Read the model definition and answer for the solid it produces. Units are mm, in the model's axes. Face numbers are marked on the shaded views. A direction names the side the tool comes from. Give positions to 0.01 mm unless a question says otherwise; leave off trailing zeros. Write each loop counter-clockwise with the first axis right and the second up, starting at its lowest first coordinate (ties: lowest second). Pieces come first, ordered by that corner, then holes. Notation, with made-up numbers: M 37,44 L 57,44 A31 cw 57,72 Z; hole C 50,30 d8. An arc over 180 degrees is marked long. Put each result on its own line as item: value.
from build123d import *

# Parameters (mm, degrees)
ESQUISSE1_R        = 4
ESQUISSE1_R_2      = 1.59999944
BOSS_EXTRU_1_DEPTH = 5


with BuildPart() as part:
    # Esquisse1 → Boss.-Extru.1 (new body)
    with BuildSketch(Plane(origin=(0, 0, 0), x_dir=(-1, 0, 0), z_dir=(0, 0, -1))):
        with BuildLine():
            Line((-8.039665, 5.193958), (-7.511682, 7.163724))
            Line((-7.511682, 7.163724), (-6.637512, 8.89434))
            Line((-6.637512, 8.89434), (-5.734358, 10.21466))
            Line((-5.734358, 10.21466), (-4.529502, 11.42329))
            Line((-4.529502, 11.42329), (-3.426544, 12.65958))
            Line((-3.426544, 12.65958), (-2.422703, 14.23997))
            Line((-2.422703, 14.23997), (-1.578115, 16.23473))
            Line((-1.578115, 16.23473), (-0.7880442, 19.27814))
            Line((-0.7880442, 19.27814), (-0.2469295, 23.26466))
            Line((-0.2469295, 23.26466), (-0.008147676, 28.26909))
            Line((-0.008147676, 28.26909), (0, 29.5))
            Line((0, 29.5), (-0.01509115, 31.16446))
            Line((-0.01509115, 31.16446), (-0.2937396, 36.23574))
            Line((-0.2937396, 36.23574), (-0.8642389, 40.10257))
            Line((-0.8642389, 40.10257), (-1.681502, 43.05889))
            Line((-1.681502, 43.05889), (-2.667923, 45.20577))
            Line((-2.667923, 45.20577), (-3.68381, 46.66188))
            Line((-3.68381, 46.66188), (-5.121313, 48.15284))
            Line((-5.121313, 48.15284), (-6.221777, 49.42276))
            Line((-6.221777, 49.42276), (-7.084233, 50.913))
            Line((-7.084233, 50.913), (-7.705722, 52.38649))
            Line((-7.705722, 52.38649), (-8.155009, 54.60259))
            Line((-8.155009, 54.60259), (-8.534575, 55.99675))
            Line((-8.534575, 55.99675), (-9.29695, 57.22417))
            Line((-9.29695, 57.22417), (-10.37847, 58.18233))
            Line((-10.37847, 58.18233), (-11.68882, 58.79123))
            Line((-11.68882, 58.79123), (-13.11856, 59))
            Line((-13.11856, 59), (-28.5, 59))
            ThreePointArc((-28.5, 59), (-28.853553391, 58.853553391), (-29, 58.5))
            Line((-29, 58.5), (-29, 54.25))
            Line((-29, 54.25), (-28.875, 54.2165))
            Line((-28.875, 54.2165), (-28.78349, 54.125))
            Line((-28.78349, 54.125), (-28.75, 54))
            Line((-28.75, 54), (-28.78349, 53.875))
            Line((-28.78349, 53.875), (-28.875, 53.78349))
            Line((-28.875, 53.78349), (-29, 53.75))
            Line((-29, 53.75), (-29.125, 53.78349))
            Line((-29.125, 53.78349), (-29.21651, 53.875))
            Line((-29.21651, 53.875), (-29.25, 54))
            Line((-29.25, 54), (-33.75, 54))
            ThreePointArc((-33.75, 54), (-34.176776695, 53.823223305), (-34, 54.25))
            Line((-34, 54.25), (-34, 58.5))
            ThreePointArc((-34, 58.5), (-34.146446609, 58.853553391), (-34.5, 59))
            Line((-34.5, 59), (-34.77157, 59))
            Line((-34.77157, 59), (-35.53694, 58.84776))
            Line((-35.53694, 58.84776), (-36.18579, 58.41422))
            Line((-36.18579, 58.41422), (-39.41421372, 55.18578628))
            ThreePointArc((-39.41421372, 55.18578628), (-39.847759129, 54.53693809), (-40, 53.77157))
            Line((-40, 53.77157), (-40, 5.228428))
            ThreePointArc((-40, 5.228428), (-39.847759811, 4.463063957), (-39.414216379, 3.814219379))
            Line((-39.414216379, 3.814219379), (-36.18579, 0.585787))
            ThreePointArc((-36.18579, 0.585787), (-35.536943679, 0.152241095), (-34.771576938, 0))
            Line((-34.771576938, 0), (-17.5, 0))
            ThreePointArc((-17.5, 0), (-17.146446609, 0.146446609), (-17, 0.5))
            Line((-17, 0.5), (-17, 4.75))
            Line((-17, 4.75), (-17.125, 4.783494))
            Line((-17.125, 4.783494), (-17.21651, 4.875))
            Line((-17.21651, 4.875), (-17.25, 5.000001))
            Line((-17.25, 5.000001), (-17.21651, 5.125001))
            Line((-17.21651, 5.125001), (-17.125, 5.216507))
            Line((-17.125, 5.216507), (-17, 5.25))
            Line((-17, 5.25), (-16.875, 5.216507))
            Line((-16.875, 5.216507), (-16.78349, 5.125001))
            Line((-16.78349, 5.125001), (-16.75, 5.000001))
            Line((-16.75, 5.000001), (-12.25, 5.000001))
            Line((-12.25, 5.000001), (-12.21651, 5.125001))
            Line((-12.21651, 5.125001), (-12.125, 5.216507))
            Line((-12.125, 5.216507), (-12, 5.25))
            Line((-12, 5.25), (-11.875, 5.216507))
            Line((-11.875, 5.216507), (-11.78349, 5.125001))
            Line((-11.78349, 5.125001), (-11.75, 5.000001))
            Line((-11.75, 5.000001), (-11.78349, 4.810393211))
            Line((-11.78349, 4.810393211), (-11.875, 4.718887211))
            Line((-11.875, 4.718887211), (-12, 4.685393211))
            Line((-12, 4.685393211), (-12, 0.500001))
            ThreePointArc((-12, 0.500001), (-11.853553098, 0.146446902), (-11.499999, 0))
            Line((-11.499999, 0), (-10.33203, 0))
            Line((-10.33203, 0), (-9.352249, 0.2564304))
            Line((-9.352249, 0.2564304), (-8.623715, 0.9599663))
            Line((-8.623715, 0.9599663), (-8.333246, 1.9302))
            Line((-8.333246, 1.9302), (-8.039665, 5.193958))
        make_face()
        with Locations((-23, 52)):
            Circle(ESQUISSE1_R, mode=Mode.SUBTRACT)
        with Locations((-23, 6.999999)):
            Circle(ESQUISSE1_R, mode=Mode.SUBTRACT)
        with Locations((-7, 29.499999)):
            Circle(ESQUISSE1_R_2, mode=Mode.SUBTRACT)
        with BuildLine():
            Line((-27.85382, 44.42105), (-25.78795, 43.4427))
            Line((-25.78795, 43.4427), (-23.54223, 43.01635))
            Line((-23.54223, 43.01635), (-21.26154, 43.1695))
            Line((-21.26154, 43.1695), (-19.09299, 43.89227))
            Line((-19.09299, 43.89227), (-17.17647, 45.13804))
            Line((-17.17647, 45.13804), (-17.04626, 45.30922))
            Line((-17.04626, 45.30922), (-17, 45.51926))
            Line((-17, 45.51926), (-17, 50.75))
            ThreePointArc((-17, 50.75), (-17.176776695, 51.176776695), (-16.75, 51))
            Line((-16.75, 51), (-12.25, 51))
            ThreePointArc((-12.25, 51), (-11.823223305, 51.176776695), (-12, 50.75))
            Line((-12, 50.75), (-12, 46.412623211))
            Line((-12, 46.412623211), (-11.9404, 46.175873211))
            Line((-11.9404, 46.175873211), (-11.7758, 45.995563211))
            Line((-11.7758, 45.995563211), (-11.54545, 45.914693211))
            Line((-11.54545, 45.914693211), (-10.113, 45.565643211))
            Line((-10.113, 45.565643211), (-8.844621, 44.813993211))
            Line((-8.844621, 44.813993211), (-7.850602, 43.725103211))
            Line((-7.850602, 43.725103211), (-7.217376, 42.393653211))
            Line((-7.217376, 42.393653211), (-7, 40.935393211))
            Line((-7, 40.935393211), (-7.619118173, 39.531113076))
            Line((-7.619118173, 39.531113076), (-8.678014173, 38.335053076))
            Line((-8.678014173, 38.335053076), (-10.060093173, 37.534003076))
            Line((-10.060093173, 37.534003076), (-12.077863173, 36.434693076))
            Line((-12.077863173, 36.434693076), (-13.732523173, 34.840353076))
            Line((-13.732523173, 34.840353076), (-14.905963173, 32.864763076))
            Line((-14.905963173, 32.864763076), (-15.514393173, 30.648993076))
            Line((-15.514393173, 30.648993076), (-15.514393173, 28.351193076))
            Line((-15.514393173, 28.351193076), (-14.905963173, 26.135413076))
            Line((-14.905963173, 26.135413076), (-13.732523173, 24.159833076))
            Line((-13.732523173, 24.159833076), (-12.077863173, 22.565493076))
            Line((-12.077863173, 22.565493076), (-10.060093173, 21.466183076))
            Line((-10.060093173, 21.466183076), (-8.678014173, 20.665133076))
            Line((-8.678014173, 20.665133076), (-7.619118173, 19.469073076))
            Line((-7.619118173, 19.469073076), (-6.991483173, 18.000093076))
            Line((-6.991483173, 18.000093076), (-7.244718, 16.45492))
            Line((-7.244718, 16.45492), (-7.954915, 15.06107))
            Line((-7.954915, 15.06107), (-9.061074, 13.95492))
            Line((-9.061074, 13.95492), (-10.45492, 13.24472))
            Line((-10.45492, 13.24472), (-12, 13))
            Line((-12, 13), (-16.0718, 13))
            Line((-16.0718, 13), (-16.27048, 13.04117))
            Line((-16.27048, 13.04117), (-16.43644, 13.1579))
            Line((-16.43644, 13.1579), (-18.19056, 14.60719))
            Line((-18.19056, 14.60719), (-20.2521, 15.57024))
            Line((-20.2521, 15.57024), (-22.48927, 15.9855))
            Line((-22.48927, 15.9855), (-24.7591, 15.82641))
            Line((-24.7591, 15.82641), (-26.91648, 15.10316))
            Line((-26.91648, 15.10316), (-28.82353, 13.86196))
            Line((-28.82353, 13.86196), (-28.95374, 13.69078))
            Line((-28.95374, 13.69078), (-29, 13.48074))
            Line((-29, 13.48074), (-29, 8.25))
            Line((-29, 8.25), (-28.875, 8.216506))
            Line((-28.875, 8.216506), (-28.78349, 8.125))
            Line((-28.78349, 8.125), (-28.75, 8))
            Line((-28.75, 8), (-28.78349, 7.875001))
            Line((-28.78349, 7.875001), (-28.875, 7.783493))
            Line((-28.875, 7.783493), (-29, 7.750001))
            Line((-29, 7.750001), (-29.125, 7.783493))
            Line((-29.125, 7.783493), (-29.21651, 7.875001))
            Line((-29.21651, 7.875001), (-29.25, 8))
            Line((-29.25, 8), (-33.75, 8))
            Line((-33.75, 8), (-33.7835, 7.875001))
            Line((-33.7835, 7.875001), (-33.875, 7.783493))
            Line((-33.875, 7.783493), (-34, 7.750001))
            Line((-34, 7.750001), (-34.125, 7.783493))
            Line((-34.125, 7.783493), (-34.21651, 7.875001))
            Line((-34.21651, 7.875001), (-34.25, 8))
            Line((-34.25, 8), (-34.21651, 8.125))
            Line((-34.21651, 8.125), (-34.125, 8.216506))
            Line((-34.125, 8.216506), (-34, 8.25))
            Line((-34, 8.25), (-34, 43.90222))
            Line((-34, 43.90222), (-33.81641, 44.73928))
            Line((-33.81641, 44.73928), (-33.29933, 45.42266))
            Line((-33.29933, 45.42266), (-32.54371, 45.8269))
            Line((-32.54371, 45.8269), (-31.68826, 45.87778))
            Line((-31.68826, 45.87778), (-29.69555, 45.34813))
            Line((-29.69555, 45.34813), (-27.85382, 44.42105))
        make_face(mode=Mode.SUBTRACT)
    extrude(amount=-BOSS_EXTRU_1_DEPTH)


solid = part.part
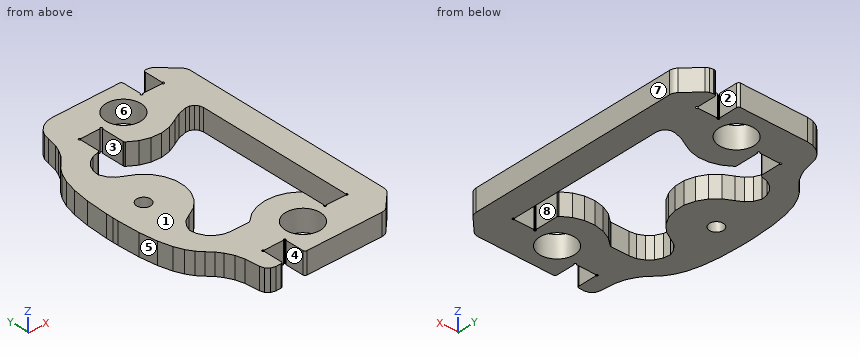
(1) Section A-A on y = 34 is taken. Determine the outline of the cut face in (x, z).
Result:
outline: M 0.17,0 L 14.23,0 L 14.23,5 L 0.17,5 Z; M 34,0 L 40,0 L 40,5 L 34,5 Z
(2) Which of the six approach directions +Z, -Z, +X, -X, +Y, -Y give full straight-line access (tool end or side, diameter ignored) to the marked faces 1, 2, 3 and 4?
Result:
face 1: +Z, +X, -X, +Y, -Y
face 2: +Z, -Z, +Y
face 3: +Z, -Z
face 4: +Z, -Z, -Y
(3) Section B-B on z = 3 is taken. Give the number of separate pieces and of enclosed holes in the cut face, and give its area (3 significant figures).
Result:
separate pieces: 1
enclosed holes: 4
area: 1,210 mm²
(4) Given pin 1 Ø1.3 at (x, z) = (15, 1.5) entering from -Y; pin 2 Ø1.3 at (y, z) = (2, 2.5) entering from -X; pin 3 Ø2 at (y, z) = (57, 2) entering from +X; pin 4 Ø5 at (x, y) = (23, 7) entering from -Z, each flat-ended and moving along its own axis, determine where each tip first touches the part or whether it passes through.
Result:
pin 1: stops at y = 5
pin 2: stops at x = 8.27
pin 3: stops at x = 38.6
pin 4: passes through
(5) For a pull along X with two mould halves and no side action, classify the marked faces 5, 6, 7 and 8 as +X half, -X half, draft (parallel to the pull), parting line (faces both ways), or undercut.
Result:
face 5: -X half
face 6: undercut
face 7: +X half
face 8: undercut
(6) Straight lines are drawn through the part: line 1 along Y through (x, z) = (23, 2.9); line 2 along X through (y, z) = (29, 4.3); line 3 along X through (y, z) = (10, 3.95). For each, find the intervals that lie inside material, in ascending order. Write a range as from..to.
Result:
line 1: y = 0..3, 11..15.95, 43.05..48, 56..59
line 2: x = 0..5.48, 8.52..15.51, 34..40
line 3: x = 5.88..20.35, 25.65..29, 34..40
(7) Section C-C on y = 27 is taken. Determine the outline of the cut face in (x, z), and give its area (3 significant figures).
Result:
outline: M 0.07,0 L 15.14,0 L 15.14,5 L 0.07,5 Z; M 34,0 L 40,0 L 40,5 L 34,5 Z
area: 105 mm²
